```python
from build123d import *

# Parameters (mm, degrees)
F0_W         = 76.2
F0_H         = 101.6
F1_DEPTH     = 38.1
F3_W         = 76.2
F3_H         = 101.6
F3_W_2       = 73.66
F3_H_2       = 99.06
F4_DEPTH     = 3.175
F5_T1_DEPTH  = 99.06
F5_T3_DEPTH  = 73.66
F5_T9_DEPTH  = 105.41
F5_T15_DEPTH = 80.01
F5_T24_DEPTH = 105.41
F5_T30_DEPTH = 80.01
F5_T39_DEPTH = 80.01
F5_T45_DEPTH = 105.41
F5_T54_DEPTH = 105.41
F5_T60_DEPTH = 80.01


# Not quite as in the source:
# - a fillet or chamfer that OpenCascade refuses, or shapes differently, is made with other operations: its cross-section is extruded or revolved along the edge and cut away or added


with BuildPart() as f1:
    # F0 (on Top) → F1 (new body)
    with BuildSketch(Plane.XY):
        Rectangle(F0_W, F0_H)
    extrude(amount=F1_DEPTH)

    # F3 (on face) → F4 (join)
    with BuildSketch(Plane(origin=(0, 0, 0), x_dir=(1, 0, 0), z_dir=(0, 0, -1))):
        Rectangle(F3_W, F3_H)
        Rectangle(F3_W_2, F3_H_2, mode=Mode.SUBTRACT)
    extrude(amount=F4_DEPTH)

    # F5: fillet of radius 2.54 on 4 edges, made by hand

    # F5_s2 → F5_t1 (cut)
    with BuildSketch(Plane.XZ.offset(-49.53)):
        with BuildLine():
            ThreePointArc((-39.37, -3.175), (-37.5739487758, -2.4310512242), (-36.83, -0.635))
            Line((-36.83, -0.635), (-36.83, -3.175))
            Line((-36.83, -3.175), (-39.37, -3.175))
        make_face()
        with BuildLine():
            ThreePointArc((39.37, -3.175), (37.5739487758, -2.4310512242), (36.83, -0.635))
            Line((36.83, -0.635), (36.83, -3.175))
            Line((36.83, -3.175), (39.37, -3.175))
        make_face()
    extrude(amount=F5_T1_DEPTH, mode=Mode.SUBTRACT)

    # F5_s4 → F5_t3 (cut)
    with BuildSketch(Plane.YZ.offset(-36.83)):
        with BuildLine():
            ThreePointArc((-52.07, -3.175), (-50.2739487758, -2.4310512242), (-49.53, -0.635))
            Line((-49.53, -0.635), (-49.53, -3.175))
            Line((-49.53, -3.175), (-52.07, -3.175))
        make_face()
        with BuildLine():
            ThreePointArc((52.07, -3.175), (50.2739487758, -2.4310512242), (49.53, -0.635))
            Line((49.53, -0.635), (49.53, -3.175))
            Line((49.53, -3.175), (52.07, -3.175))
        make_face()
    extrude(amount=F5_T3_DEPTH, mode=Mode.SUBTRACT)


with BuildPart() as f5_tool7:
    # F5_s8 → F5_t9 (new body)
    with BuildSketch(Plane.XZ.offset(-55.88)):
        with BuildLine():
            ThreePointArc((-39.37, -3.175), (-37.5739487758, -2.4310512242), (-36.83, -0.635))
            Line((-36.83, -0.635), (-36.83, -3.175))
            Line((-36.83, -3.175), (-39.37, -3.175))
        make_face()
    extrude(amount=F5_T9_DEPTH)

    split(bisect_by=Plane.XZ.offset(-49.53), keep=Keep.BOTTOM)

    split(bisect_by=Plane.YZ.offset(-38.1), keep=Keep.TOP)

    split(bisect_by=Plane.XZ.offset(-50.8), keep=Keep.TOP)


with BuildPart() as f5_tool13:
    # F5_s14 → F5_t15 (new body)
    with BuildSketch(Plane.YZ.offset(36.83)):
        with BuildLine():
            ThreePointArc((52.07, -3.175), (50.2739487758, -2.4310512242), (49.53, -0.635))
            Line((49.53, -0.635), (49.53, -3.175))
            Line((49.53, -3.175), (52.07, -3.175))
        make_face()
    extrude(amount=-F5_T15_DEPTH)

    split(bisect_by=Plane.YZ.offset(-36.83), keep=Keep.BOTTOM)

    split(bisect_by=Plane.YZ.offset(-38.1), keep=Keep.TOP)

    split(bisect_by=Plane.XZ.offset(-50.8), keep=Keep.TOP)


with BuildPart() as f5_tool7_1:
    add(f5_tool7.part)

    # F5_t19: intersect F5_tool13
    add(f5_tool13.part, mode=Mode.INTERSECT)


with BuildPart() as f1_1:
    add(f1.part)

    # F5_t5: cut F5_tool7
    add(f5_tool7_1.part, mode=Mode.SUBTRACT)


with BuildPart() as f5_tool22:
    # F5_s23 → F5_t24 (new body)
    with BuildSketch(Plane.XZ.offset(-49.53)):
        with BuildLine():
            ThreePointArc((-39.37, -3.175), (-37.5739487758, -2.4310512242), (-36.83, -0.635))
            Line((-36.83, -0.635), (-36.83, -3.175))
            Line((-36.83, -3.175), (-39.37, -3.175))
        make_face()
    extrude(amount=F5_T24_DEPTH)

    split(bisect_by=Plane.XZ.offset(49.53), keep=Keep.TOP)

    split(bisect_by=Plane.YZ.offset(-38.1), keep=Keep.TOP)

    split(bisect_by=Plane.XZ.offset(50.8), keep=Keep.BOTTOM)


with BuildPart() as f5_tool28:
    # F5_s29 → F5_t30 (new body)
    with BuildSketch(Plane.YZ.offset(-43.18)):
        with BuildLine():
            ThreePointArc((-52.07, -3.175), (-50.2739487758, -2.4310512242), (-49.53, -0.635))
            Line((-49.53, -0.635), (-49.53, -3.175))
            Line((-49.53, -3.175), (-52.07, -3.175))
        make_face()
    extrude(amount=F5_T30_DEPTH)

    split(bisect_by=Plane.YZ.offset(-36.83), keep=Keep.BOTTOM)

    split(bisect_by=Plane.YZ.offset(-38.1), keep=Keep.TOP)

    split(bisect_by=Plane.XZ.offset(50.8), keep=Keep.BOTTOM)


with BuildPart() as f5_tool22_1:
    add(f5_tool22.part)

    # F5_t34: intersect F5_tool28
    add(f5_tool28.part, mode=Mode.INTERSECT)


with BuildPart() as f1_2:
    add(f1_1.part)

    # F5_t20: cut F5_tool22
    add(f5_tool22_1.part, mode=Mode.SUBTRACT)


with BuildPart() as f5_tool37:
    # F5_s38 → F5_t39 (new body)
    with BuildSketch(Plane.YZ.offset(-36.83)):
        with BuildLine():
            ThreePointArc((-52.07, -3.175), (-50.2739487758, -2.4310512242), (-49.53, -0.635))
            Line((-49.53, -0.635), (-49.53, -3.175))
            Line((-49.53, -3.175), (-52.07, -3.175))
        make_face()
    extrude(amount=F5_T39_DEPTH)

    split(bisect_by=Plane.YZ.offset(38.1), keep=Keep.BOTTOM)

    split(bisect_by=Plane.YZ.offset(36.83), keep=Keep.TOP)

    split(bisect_by=Plane.XZ.offset(50.8), keep=Keep.BOTTOM)


with BuildPart() as f5_tool43:
    # F5_s44 → F5_t45 (new body)
    with BuildSketch(Plane.XZ.offset(55.88)):
        with BuildLine():
            ThreePointArc((39.37, -3.175), (37.5739487758, -2.4310512242), (36.83, -0.635))
            Line((36.83, -0.635), (36.83, -3.175))
            Line((36.83, -3.175), (39.37, -3.175))
        make_face()
    extrude(amount=-F5_T45_DEPTH)

    split(bisect_by=Plane.YZ.offset(38.1), keep=Keep.BOTTOM)

    split(bisect_by=Plane.XZ.offset(49.53), keep=Keep.TOP)

    split(bisect_by=Plane.XZ.offset(50.8), keep=Keep.BOTTOM)


with BuildPart() as f5_tool37_1:
    add(f5_tool37.part)

    # F5_t49: intersect F5_tool43
    add(f5_tool43.part, mode=Mode.INTERSECT)


with BuildPart() as f1_3:
    add(f1_2.part)

    # F5_t35: cut F5_tool37
    add(f5_tool37_1.part, mode=Mode.SUBTRACT)


with BuildPart() as f5_tool52:
    # F5_s53 → F5_t54 (new body)
    with BuildSketch(Plane.XZ.offset(49.53)):
        with BuildLine():
            ThreePointArc((39.37, -3.175), (37.5739487758, -2.4310512242), (36.83, -0.635))
            Line((36.83, -0.635), (36.83, -3.175))
            Line((36.83, -3.175), (39.37, -3.175))
        make_face()
    extrude(amount=-F5_T54_DEPTH)

    split(bisect_by=Plane.YZ.offset(38.1), keep=Keep.BOTTOM)

    split(bisect_by=Plane.XZ.offset(-49.53), keep=Keep.BOTTOM)

    split(bisect_by=Plane.XZ.offset(-50.8), keep=Keep.TOP)


with BuildPart() as f5_tool58:
    # F5_s59 → F5_t60 (new body)
    with BuildSketch(Plane.YZ.offset(43.18)):
        with BuildLine():
            ThreePointArc((52.07, -3.175), (50.2739487758, -2.4310512242), (49.53, -0.635))
            Line((49.53, -0.635), (49.53, -3.175))
            Line((49.53, -3.175), (52.07, -3.175))
        make_face()
    extrude(amount=-F5_T60_DEPTH)

    split(bisect_by=Plane.YZ.offset(38.1), keep=Keep.BOTTOM)

    split(bisect_by=Plane.YZ.offset(36.83), keep=Keep.TOP)

    split(bisect_by=Plane.XZ.offset(-50.8), keep=Keep.TOP)


with BuildPart() as f5_tool52_1:
    add(f5_tool52.part)

    # F5_t64: intersect F5_tool58
    add(f5_tool58.part, mode=Mode.INTERSECT)


with BuildPart() as f1_4:
    add(f1_3.part)

    # F5_t50: cut F5_tool52
    add(f5_tool52_1.part, mode=Mode.SUBTRACT)


solid = f1_4.part
```
Work out the finished part from the listing and answer in its coordinate system (mm). A direction names the side the tool comes from. Give positions to 0.01 mm unless a question says otherwise; leave off trailing zeros. Order: outer loops, then holes, each group sorted by start corner. A loop starts at its lowest first (then second) coordinate and runs counter-clockwise, first axis right, second up. Notation, with made-up numbers: (41.5, 29) - (66.5, 29) arc R18 ccw to (66.5, 42) - close; hole circle Ø3 at (41.5, -33.75). An arc over 180 degrees is marked (long way). One line per item, written item: value. Start each with the question number.
1. Section B-B, the plane x = -21 is taken. Write down the section's boundary in (y, z) (3 decimals).
2. This flat-tipped pin is pushed along its axis until it touches: pin 1 Ø3 at (x, y) = (22.5, 11) entering from -Z. Where does it stop, or does it pass through?
3. For a pull along X with two mould halves and no side action, classify faces 3 (the face through (37.18, -0.71, -1.92)), 4 (the face through (38.1, 1, 18)), 5 (the face through (-1, 50.8, 18)) as released by +X, released by -X, zero draft, split by the parting line, or undercut.
4. Which of the six approach directions +Z, -Z, +X, -X, +Y, -Y give full straight-line access (tool end or side, diameter ignored) to faces 1 (the face through (-37.18, 0.71, -1.92)), 2 (the face through (-1, 1, 38.1))?
5. Section A-A, the plane y = -4 is taken. Write down the section's boundary in (x, z) (3 decimals).
6. Consider line 1 (Z direction, x = 32, y = 32). Determine where the line is inside the solid, lowest interval first.
Filled sheet:
1. outline: (-50.8, -2.835) arc R2.54 ccw to (-49.53, -0.635) - (-49.53, 0) - (49.53, 0) - (49.53, -0.635) arc R2.54 ccw to (50.8, -2.835) - (50.8, 38.1) - (-50.8, 38.1) - close
2. pin 1: z = 0
3. face 3: undercut
3. face 4: released by +X
3. face 5: zero draft
4. face 1: -Z
4. face 2: +Z, +X, -X, +Y, -Y
5. outline: (-38.1, -2.835) arc R2.54 ccw to (-36.83, -0.635) - (-36.83, 0) - (36.83, 0) - (36.83, -0.635) arc R2.54 ccw to (38.1, -2.835) - (38.1, 38.1) - (-38.1, 38.1) - close
6. line 1: 0 to 38.1
